Check sheet for the modelled part. Datum: model origin and axes. Units: mm. Coordinates: 2 decimals unless noted, no trailing zeros. Order: outer loops, then holes, each group sorted by start corner. A loop starts at its lowest first (then second) coordinate and runs counter-clockwise, first axis right, second up.
1. Cross-section at A-A (x = 2.5). Enter the section's corners in (y, z), then the cut area to 3 significant figures.
2. Gauge pin test, flat end, axial feed: pin 1 Ø3 at (x, y) = (0.5, 2) entering from +Z. Record the tip position at first contact, or that the pin passes through.
3. Draft check along Y on faces 1 (the flat face through (2, 5, -2)), 2 (the flat face through (2, 0, -2)), 3 (the flat face through (4, 3, -5)), 4 (the cylindrical face through (1.5, 2.5, -2.5)). Enter one of: released by +Y, released by -Y, zero draft, split by the parting line, or undercut.
4. Thickness scan on line 1 (Y direction, x = 2.5, z = -1.6); line 2 (X direction, y = 3.05, z = -2.65); line 3 (X direction, y = 3.3, z = -4.3). Record the ranges inside material, lowest first.
5. Cross-section at C-C (z = -3). Enter the section's corners in (x, y), then the cut area to 3 significant figures.
```python
from build123d import *

# Parameters (mm, degrees)
SKETCH_1_W          = 5
SKETCH_1_H          = 5
EXTRUDE_1_DEPTH     = 5
SKETCH_3_R          = 1
CUT_EXTRUDE_1_DEPTH = 5


with BuildPart() as part:
    # 草图1 → 凸台-拉伸1 (new body)
    with BuildSketch(Plane.XY):
        with Locations((2.5, 2.5)):
            Rectangle(SKETCH_1_W, SKETCH_1_H)
    extrude(amount=-EXTRUDE_1_DEPTH)

    # 草图3 → 切除-拉伸1 (cut)
    with BuildSketch(Plane.XY):
        with Locations((2.5, 2.5)):
            Circle(SKETCH_3_R)
    extrude(amount=-CUT_EXTRUDE_1_DEPTH, mode=Mode.SUBTRACT)


solid = part.part
```
Data:
1. outline: (0, -5) - (1.5, -5) - (1.5, 0) - (0, 0) - close; (3.5, -5) - (5, -5) - (5, 0) - (3.5, 0) - close
1. area: 15.0 mm2
2. pin 1: stops at z = 0
3. face 1: released by +Y
3. face 2: released by -Y
3. face 3: zero draft
3. face 4: undercut
4. line 1: y = 0 to 1.5, 3.5 to 5
4. line 2: x = 0 to 1.66, 3.34 to 5
4. line 3: x = 0 to 1.9, 3.1 to 5
5. outline: (0, 0) - (5, 0) - (5, 5) - (0, 5) - close; hole circle Ø2 at (2.5, 2.5)
5. area: 21.9 mm2
